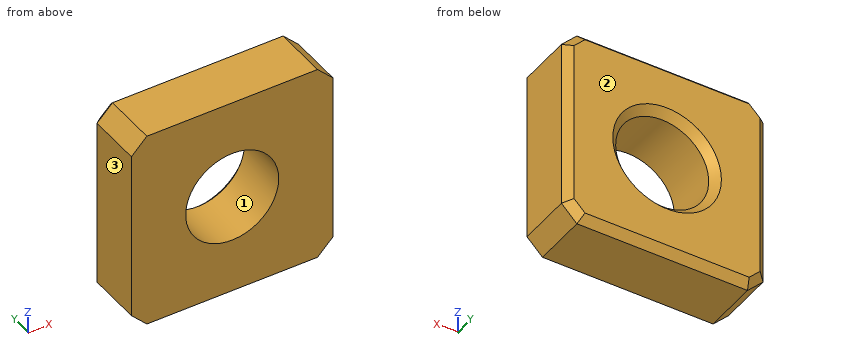
```python
from build123d import *

# Parameters (mm, degrees)
SKETCH1_W           = 13
SKETCH1_H           = 13
SKETCH1_R           = 3
BOSS_EXTRUDE1_DEPTH = 4
CHAMFER1_SIZE       = 1
CHAMFER3_SIZE       = 0.5


with BuildPart() as part:
    # Sketch1 → Boss-Extrude1 (new body)
    with BuildSketch(Plane(origin=(0, 0, 0), x_dir=(1, 0, 0), z_dir=(0, 1, 0))):
        Rectangle(SKETCH1_W, SKETCH1_H)
        Circle(SKETCH1_R, mode=Mode.SUBTRACT)
    extrude(amount=BOSS_EXTRUDE1_DEPTH)

    # Chamfer1
    chamfer1_edges = [part.edges().sort_by_distance(p)[0] for p in [
        (6.5, 2, 6.5),
        (-6.5, 2, 6.5),
        (-6.5, 2, -6.5),
        (6.5, 2, -6.5),
    ]]
    chamfer(chamfer1_edges, length=CHAMFER1_SIZE)

    # Chamfer3
    chamfer3_edges = [part.edges().sort_by_distance(p)[0] for p in [
        (-3, 4, 0),
        (-6.5, 4, 0),
        (0, 4, -6.5),
        (6.5, 4, 0),
        (0, 4, 6.5),
        (6, 4, 6),
        (6, 4, -6),
        (-6, 4, 6),
        (-6, 4, -6),
    ]]
    chamfer(chamfer3_edges, length=CHAMFER3_SIZE)


solid = part.part
```
Input: part model. Units: mm. Frame: model coordinates. Face numbers are marked on the shaded views. Coordinates: 2 decimals unless noted, no trailing zeros. Write each loop counter-clockwise with the first axis right and the second up, starting at its lowest first coordinate (ties: lowest second). Pieces come first, ordered by that corner, then holes. Notation, with made-up numbers: (84.25, 41) -> (117.25, 41) arc R33 cw to (117.25, 79) -> close; hole circle Ø8 at (17, -4.5). An arc over 180 degrees is marked (long way). Write each question's results on one line, items separated by ' | '.
Item 1: Section query A-A on z = 0. Return loops of the section in (x, y), plus the area to 3 significant figures.
Conclusion:
outline: (-6.5, 0) -> (-3, 0) -> (-3, 3.5) -> (-3.5, 4) -> (-6, 4) -> (-6.5, 3.5) -> close; (3, 0) -> (6.5, 0) -> (6.5, 3.5) -> (6, 4) -> (3.5, 4) -> (3, 3.5) -> close | area: 27.5 mm^2
Item 2: Mould query, pull axis X, two halves, no side actions, for the marked faces 1, 2 and 3. Classes: +X half, -X half, draft (parallel to the pull), parting line (faces both ways), or undercut.
Conclusion:
face 1: undercut | face 2: draft | face 3: -X half
Item 3: Section query C-C on y = 3.25. Return loops of the section in (x, z).
Conclusion:
outline: (-6.5, -5.5) -> (-5.5, -6.5) -> (5.5, -6.5) -> (6.5, -5.5) -> (6.5, 5.5) -> (5.5, 6.5) -> (-5.5, 6.5) -> (-6.5, 5.5) -> close; hole circle Ø6 at (0, 0)
Item 4: Pin query (flat end, axial travel): pin 1 Ø2 at (x, z) = (1, -0.5) entering from -Y. Return the tip coordinate at first contact, or that it passes through.
Conclusion:
pin 1: passes through
Item 5: Material intervals for probe 1 along X at (y, z) = (2.7, 0); probe 2 along X at (y, z) = (3.85, -2), sorted ascending.
Conclusion:
probe 1: x = -6.5 to -3, 3 to 6.5 | probe 2: x = -6.15 to -2.69, 2.69 to 6.15
Item 6: Section query B-B on x = 0. Return loops of the section in (y, z), plus the area to 3 significant figures.
Conclusion:
outline: (0, -6.5) -> (3.5, -6.5) -> (4, -6) -> (4, -3.5) -> (3.5, -3) -> (0, -3) -> close; (0, 3) -> (3.5, 3) -> (4, 3.5) -> (4, 6) -> (3.5, 6.5) -> (0, 6.5) -> close | area: 27.5 mm^2
